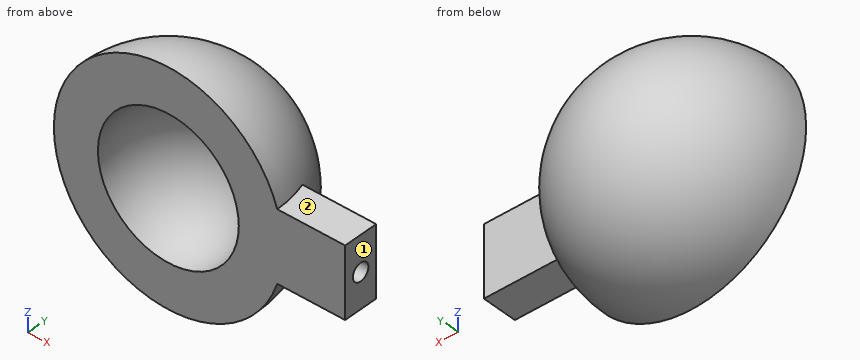
```python
from build123d import *

# Parameters (mm, degrees)
BOSS_EXTRUDE1_DEPTH = 2
SKETCH3_R           = 0.5
CUT_EXTRUDE1_DEPTH  = 2


with BuildPart() as part:
    # Sketch1 → Revolve1 (revolve)
    with BuildSketch(Plane.XY):
        with BuildLine():
            ThreePointArc((-4, 0), (-2.828427125, 2.828427125), (0, 4))
            Line((0, 4), (0, 4.973305283))
            Line((0, 4.973305283), (0, 6.5))
            ThreePointArc((0, 6.5), (-4.596194078, 4.596194078), (-6.5, 0))
            Line((-6.5, 0), (-4, 0))
        make_face()
    revolve(axis=Axis((0, 0, 0), (0, 1, 0)))

    # Sketch2 → Boss-Extrude1 (add)
    with BuildSketch(Plane.XZ):
        with BuildLine():
            Line((10.037634205, 2), (3.464101615, 2))
            ThreePointArc((3.464101615, 2), (3.863703305, 1.03527618), (4, 0))
            ThreePointArc((4, 0), (3.863703305, -1.03527618), (3.464101615, -2))
            Line((3.464101615, -2), (10.037634205, -2))
            Line((10.037634205, -2), (10.037634205, 0))
            Line((10.037634205, 0), (10.037634205, 2))
        make_face()
    extrude(amount=-BOSS_EXTRUDE1_DEPTH)

    # Sketch3 → Cut-Extrude1 (cut)
    with BuildSketch(Plane(origin=(10.037634205, 0, 0), x_dir=(0, 0, -1), z_dir=(1, 0, 0))):
        with Locations((0, 1)):
            Circle(SKETCH3_R)
    extrude(amount=-CUT_EXTRUDE1_DEPTH, mode=Mode.SUBTRACT)


solid = part.part
```
For this review, take the finished solid that the model builds, in its own axes (mm). Face numbers are marked on the shaded views. Coordinates: 2 decimals unless noted, no trailing zeros. Loops run counter-clockwise (first coordinate to the right, second up) from the corner with the lowest first, then second, coordinate; pieces in that order, holes last. Notation, with made-up numbers: (82.25, 53.25) -> (113.25, 53.25) arc R17 ccw to (113.25, 69.25) -> close; hole circle Ø1 at (-37, -32). An arc over 180 degrees is marked (long way). Return JSON: item names as keys, results as strings. Group by question number.
(1) Consider section C-C, the plane x = -3.5. Give the boundary of the cut face in (y, z), plus the area to 3 significant figures.
(2) Consider section B-B, the plane y = 1. Give the boundary of the cut face in (x, z), plus the area to 3 significant figures.
(3) To check wall thickness, follow L1, parallel to Y at x = 9.5, z = 0; L2, parallel to Z at x = 2, y = 2.5; L3, parallel to X at y = 2.75, z = -1. State the ranges of each line that lie inside material, in increasing order.
(4) Mouldability with a two-part tool opening along X and no side actions: class the marked faces 1 and 2 as pulls with the +X half, pulls with the -X half, needs draft (parallel to the pull), parting line crosses it, or undercut.
(5) Consider section D-D, the plane y = 5. Give the boundary of the cut face in (x, z), plus the area to 3 significant figures.
(6) For pin 1 Ø6 at (x, z) = (-2.5, -1) entering from +Y; pin 2 Ø4.5 at (x, z) = (7.5, 0) entering from +Y; pin 3 Ø1.5 at (x, y) = (-1.5, 4.5) entering from +Z; pin 4 Ø0.6 at (x, y) = (8.5, 1) entering from -Z, all flat-tipped, find the tip position at first contact; note any pin that passes through.
(7) Consider section A-A, the plane z = 0. Give the boundary of the cut face in (x, y).
Results below:
{
 "1": {"outline": "(0, -5.48) arc R5.48 ccw to (0, 5.48) -> (0, 1.94) arc R1.94 cw to (0, -1.94) -> close", "area": "41.2 mm2"},
 "2": {"outline": "(6.1, -2) -> (10.04, -2) -> (10.04, -0.5) -> (8.04, -0.5) -> (8.04, 0.5) -> (10.04, 0.5) -> (10.04, 2) -> (6.1, 2) arc R6.42 ccw (long way) to start; hole circle Ø7.75 at (0, 0)", "area": "95.3 mm2"},
 "3": {"L1": "y = 0 to 0.5, 1.5 to 2", "L2": "z = -5.66 to -2.4, 2.4 to 5.66", "L3": "x = -5.8 to -2.73, 2.73 to 5.8"},
 "4": {"face 1": "pulls with the +X half", "face 2": "needs draft"},
 "5": {"outline": "circle Ø8.31 at (0, 0)", "area": "54.2 mm2"},
 "6": {"pin 1": "stops at y = 6.5", "pin 2": "stops at y = 3.83", "pin 3": "stops at z = 5.13", "pin 4": "stops at z = -2"},
 "7": {"outline": "(-6.5, 0) -> (-4, 0) arc R4 cw to (4, 0) -> (10.04, 0) -> (10.04, 0.5) -> (8.04, 0.5) -> (8.04, 1.5) -> (10.04, 1.5) -> (10.04, 2) -> (6.18, 2) arc R6.5 ccw to start"}
}
